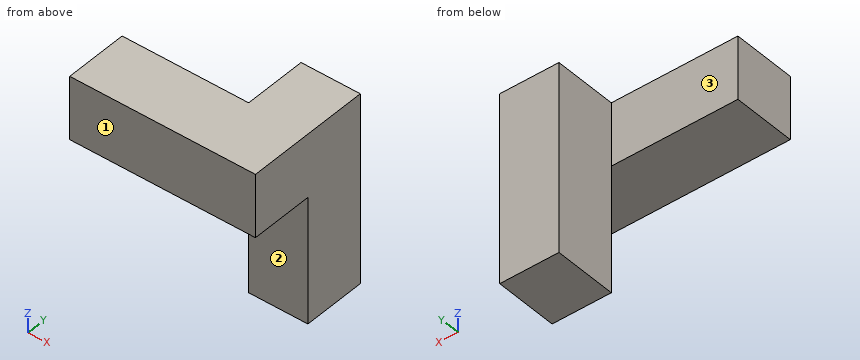
```python
from build123d import *

# Parameters (mm, degrees)
F0_W     = 17.837725
F0_H     = 19.05
F1_DEPTH = 19.05
F2_W     = 17.837725
F2_H     = 19.05
F2_W_2   = 19.05
F3_DEPTH = 19.05


with BuildPart() as f1:
    # F0 (on Front) → F1 (new body)
    with BuildSketch(Plane.XZ):
        with Locations((42.629033, 37.424813)):
            Rectangle(F0_W, F0_H)
        with Locations((42.629033, 18.374813)):
            Rectangle(F0_W, F0_H)
        with Locations((42.629033, -0.675187)):
            Rectangle(F0_W, F0_H)
    extrude(amount=F1_DEPTH)

    # F2 (on face) → F3 (join)
    with BuildSketch(Plane.XZ.offset(19.05)):
        with Locations((42.629033, 37.424813)):
            Rectangle(F2_W, F2_H)
        with Locations((24.185171, 37.424813)):
            Rectangle(F2_W_2, F2_H)
        with Locations((5.135171, 37.424813)):
            Rectangle(F2_W_2, F2_H)
    extrude(amount=F3_DEPTH)


solid = f1.part
```
The model under review builds one solid part; all positions refer to its coordinate system, in mm. Face numbers are marked on the shaded views. A direction names the side the tool comes from. Give positions to 0.01 mm unless a question says otherwise; leave off trailing zeros. Write each loop counter-clockwise with the first axis right and the second up, starting at its lowest first coordinate (ties: lowest second). Pieces come first, ordered by that corner, then holes. Notation, with made-up numbers: M -14,-15.75 L 27,-15.75 A26 ccw 27,-0.75 Z; hole C -11.5,27 d9. An arc over 180 degrees is marked long. Write item = value, one per line. Start each with the question number.
Q1. We need section D-D (y = -3.5). State the section outline as (x, z) points.
Q2. For line 1 (X direction, y = -11.5, z = 13); line 2 (Y direction, x = 19.5, z = 28); line 3 (Z direction, x = 22, y = -24), list the stretches that pass through material, from the lowest coordinate up.
Q3. We need section A-A (x = 47). State the section outline as (y, z) points, plus the area to 3 significant figures.
Q4. We need section B-B (z = 38). State the section outline as (x, y) points.
Q5. Clearance check with flat-ended pins moving along their axes: pin 1 (19.5 mm diameter, centred on x = 46, z = 4.5, fed in from -Y); pin 2 (12 mm diameter, centred on x = 25, y = -26, fed in from -Z); pin 3 (9.5 mm diameter, centred on x = 16.5, z = 42, fed in from +Y). State where each tip first meets the part, or that it passes through.
Q6. We need section C-C (y = -30). State the section outline as (x, z) points, plus the area to 3 significant figures.
Q7. Machinability: for the marked faces 1, 2 and 3, which of the approach directions +Z, -Z, +X, -X, +Y, -Y give a long, thin tool a straight path to every point of the face, cutting with its end or side? Answer none if there is none.
Result set:
q1.outline = M 33.71,-10.2 L 51.55,-10.2 L 51.55,46.95 L 33.71,46.95 Z
q2.line_1 = 33.71 to 51.55
q2.line_2 = -38.1 to -19.05
q2.line_3 = 27.9 to 46.95
q3.outline = M -38.1,27.9 L -19.05,27.9 L -19.05,-10.2 L 0,-10.2 L 0,46.95 L -38.1,46.95 Z
q3.area = 1,450 mm2
q4.outline = M -4.39,-38.1 L 51.55,-38.1 L 51.55,0 L 33.71,0 L 33.71,-19.05 L -4.39,-19.05 Z
q5.pin_1 = -19.05
q5.pin_2 = 27.9
q5.pin_3 = -19.05
q6.outline = M -4.39,27.9 L 51.55,27.9 L 51.55,46.95 L -4.39,46.95 Z
q6.area = 1,070 mm2
q7.face_1 = +Z, -Z, +X, -X, -Y
q7.face_2 = -Z, +X, -X, -Y
q7.face_3 = +Z, -Z, -X, +Y
